Autodesk Inventor part; units mm, degrees
ref_plane "YZ Plane" through (0, 0, 0) normal (1, 0, 0) x (0, 1, 0)
ref_plane "XZ Plane" through (0, 0, 0) normal (0, 1, 0) x (-1, 0, 0)
ref_plane "XY Plane" through (0, 0, 0) normal (0, 0, 1) x (1, 0, 0)
sketch "Szkic1" plane through (0, 0, 0) normal (0, 1, 0) x (-1, 0, 0)
  line L0 (-30, 37.5) -> (30, 37.5)
  line L1 (30, 37.5) -> (30, -37.5)
  line L2 (30, -37.5) -> (-30, -37.5)
  line L3 (-30, -37.5) -> (-30, 37.5)
  line L4 (-30, 37.5) -> (30, -37.5) construction
  line L5 (30, 37.5) -> (-30, -37.5) construction
  point P0 (0, 0)
  dimension "d0" = 60
  dimension "d1" = 75
extrude "Wyciągnięcie proste1" add sketch "Szkic1" along normal blind 8
sketch "Szkic2" plane through (0, 8, 0) normal (0, 1, 0) x (1, 0, 0)
  line L0 (-30, -37.5) -> (30, -37.5)
  line L1 (0, -37.5) -> (0, -2.5)
  circle A0 centre (0, -2.5) radius 20
  point P0 (0, 0)
  dimension "d4" = 35
  dimension "d5" = 40
extrude "Wyciągnięcie proste2" cut sketch "Szkic2" against normal blind 2
sketch "Szkic3" plane through (0, 6, 2.5) normal (0, 1, 0) x (1, 0, 0)
  circle A0 centre (0, 0) radius 20
  circle A1 centre (0, 0) radius 5
  point P0 (0, 2.5)
  dimension "d8" = 10
extrude "Wyciągnięcie proste3" cut sketch "Szkic3" against normal up to next contours A1
sketch "Szkic4" plane through (0, 0, 0) normal (0, -1, 0) x (1, 0, 0)
  circle A0 centre (0, 2.5) radius 5
  circle A1 centre (0, 2.5) radius 15
  point P0 (0, 0)
  dimension "d11" = 30
extrude "Wyciągnięcie proste4" cut sketch "Szkic4" against normal up to next
properties part number "Uchwyt silnika krokowego osi Z - płaski"
Check sheet for the modelled part. Datum: model origin and axes. Units: mm. A direction names the side the tool comes from. Give positions to 0.01 mm unless a question says otherwise; leave off trailing zeros. Order: outer loops, then holes, each group sorted by start corner. A loop starts at its lowest first (then second) coordinate and runs counter-clockwise, first axis right, second up. Notation, with made-up numbers: M 68.25,1 L 98.25,1 A25 cw 98.25,19 Z; hole C 2,-37.75 d7. An arc over 180 degrees is marked long. Answer as CSV lines item,"result". Start each with the question number.
Item 1: Cross-section at B-B on x = 0. Enter the section's corners in (y, z).
Item 2: Cross-section at C-C on y = 3.25. Enter the section's corners in (x, z), plus the area to 3 significant figures.
Item 3: Mould release check, pull along Z, two halves, no side actions. Record for faces 1 (the face through (-4.336, 7.014, 22.024)), 2 (the face through (0, 4, -37.5)), 3 (the face through (30, 4, -1)): +Z half, -Z half, draft (parallel to the pull), parting line (faces both ways), or undercut.
Item 4: Gauge pin test, flat end, axial feed: P1, Ø12, axis at x = 8, z = -2.5, coming from the +Y side. Record the tip position at first contact, or that the pin passes through.
Item 5: Thickness scan on line 1 (Z direction, x = 0, y = 1.8); line 2 (Z direction, x = 0, y = 7.05); line 3 (Y direction, x = -4.5, z = -16). Record the ranges inside material, lowest first. Write a range as [from, to].
Item 6: Tool access check on faces 4 (the face through (0, 4, 37.5)), 5 (the face through (2.9, 6, -12.4)). Record the directions out of +Z, -Z, +X, -X, +Y, -Y that give a thin tool (end or side, any length) a straight path to the whole face; none if there is none.
Item 7: Cross-section at A-A on z = 2.5. Enter the section's corners in (x, y).
Established:
1,outline,"M 0,-37.5 L 8,-37.5 L 8,-17.5 L 6,-17.5 L 6,-12.5 L 0,-12.5 Z; M 0,17.5 L 6,17.5 L 6,22.5 L 8,22.5 L 8,37.5 L 0,37.5 Z"
2,outline,"M -30,-37.5 L 30,-37.5 L 30,37.5 L -30,37.5 Z; hole C 0,2.5 d30"
2,area,"3,790 mm^2"
3,face 1,"undercut"
3,face 2,"-Z half"
3,face 3,"draft"
4,P1,"stops at y = 6"
5,line 1,"z = [-37.5, -12.5], [17.5, 37.5]"
5,line 2,"z = [-37.5, -17.5], [22.5, 37.5]"
5,line 3,"y = [0, 6]"
6,face 4,"+Z, +X, -X, +Y, -Y"
6,face 5,"+Y"
7,outline,"M -30,0 L -15,0 L -15,6 L -20,6 L -20,8 L -30,8 Z; M 15,0 L 30,0 L 30,8 L 20,8 L 20,6 L 15,6 Z"
